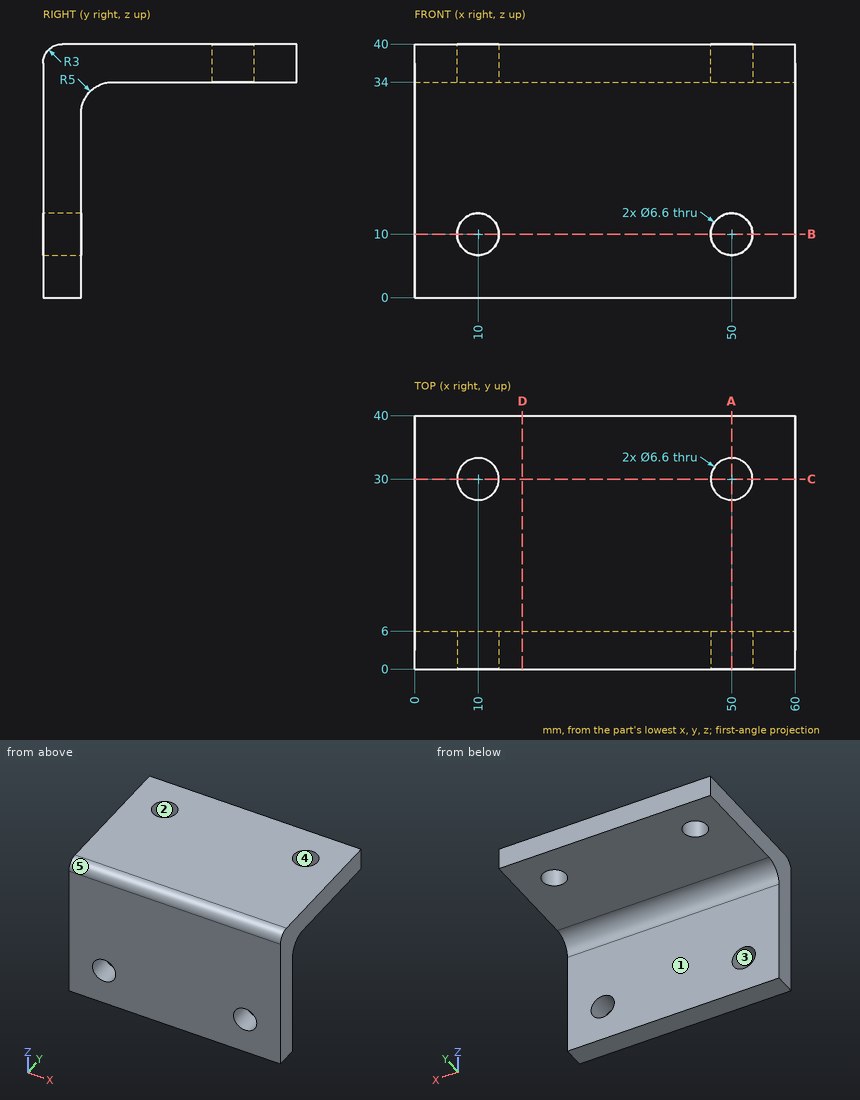
Part print with two shaded views. Sizes in mm from the minimum x, y, z corner. A direction names the side the tool comes from. Round coordinates to 2 decimals unless told otherwise and drop trailing zeros. Loops run counter-clockwise (first coordinate to the right, second up) from the corner with the lowest first, then second, coordinate; pieces in that order, holes last.
1. Slice it at B-B (z = 10). Give the cut face in (x, y).
Solutions:
outline: (0, 0) - (6.7, 0) - (6.7, 6) - (0, 6) - close; (13.3, 0) - (46.7, 0) - (46.7, 6) - (13.3, 6) - close; (53.3, 0) - (60, 0) - (60, 6) - (53.3, 6) - close
2. Two-plate mould, pull along Z, no slides. Class the marked faces 3, 4 and 5: pulls with the +Z half, pulls with the -Z half, needs draft (parallel to the pull), parting line crosses it, or undercut.
Solutions:
face 3: undercut
face 4: needs draft
face 5: pulls with the +Z half
3. Flat gauge pins, fed straight in: pin 1 (8.5 mm diameter, centred on x = 50, y = 30, fed in from -Z); pin 2 (6 mm diameter, centred on x = 50, z = 10, fed in from -Y). Where does each tip first touch, or does it go through?
Solutions:
pin 1: stops at z = 34
pin 2: passes through
4. Slice it at A-A (x = 50). Give the cut face in (y, z).
Solutions:
outline: (0, 0) - (6, 0) - (6, 6.7) - (0, 6.7) - close; (0, 13.3) - (6, 13.3) - (6, 29) arc R5 cw to (11, 34) - (26.7, 34) - (26.7, 40) - (3, 40) arc R3 ccw to (0, 37) - close; (33.3, 34) - (40, 34) - (40, 40) - (33.3, 40) - close
5. Drill centre lines: line 1 along X through (y, z) = (4.05, 10); line 2 along Z through (x, y) = (27.5, 14); line 3 along Z through (x, y) = (50, 2). Where is each one in solid material? Low to high.
Solutions:
line 1: x = 0 to 6.7, 13.3 to 46.7, 53.3 to 60
line 2: z = 34 to 40
line 3: z = 0 to 6.7, 13.3 to 39.83
6. Slice it at D-D (x = 17). Give the cut face in (y, z).
Solutions:
outline: (0, 0) - (6, 0) - (6, 29) arc R5 cw to (11, 34) - (40, 34) - (40, 40) - (3, 40) arc R3 ccw to (0, 37) - close
7. 3-axis set-ups, long thin cutter, end or side, ignore diameter. For the marked faces 1 and 2: which of +Z, -Z, +X, -X, +Y, -Y reach the whole face in a straight line?
Solutions:
face 1: -Z, +X, -X, +Y
face 2: +Z, -Z
8. Slice it at C-C (y = 30). Give the cut face in (x, z).
Solutions:
outline: (0, 34) - (6.7, 34) - (6.7, 40) - (0, 40) - close; (13.3, 34) - (46.7, 34) - (46.7, 40) - (13.3, 40) - close; (53.3, 34) - (60, 34) - (60, 40) - (53.3, 40) - close
